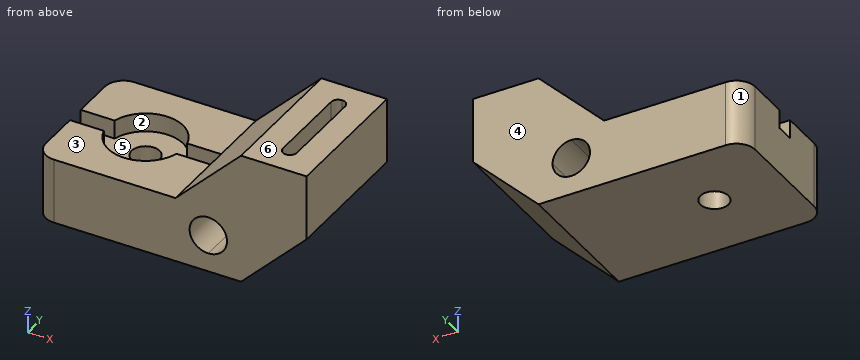
from build123d import *

# Parameters (mm, degrees)
F1_DEPTH = 76.2
F3_DEPTH = 177.8
F5_DEPTH = 27.94
F7_DEPTH = 10.16
F8_R     = 7.62
F9_DEPTH = 152.4
F10_R    = 10.16


with BuildPart() as f1:
    # F0 (on Front) → F1 (new body)
    with BuildSketch(Plane.XZ):
        Polygon((0, 35.56), (0, 0), (111.76, 0), (147.32, 35.56), (147.32, 71.12), (111.76, 71.12), (76.2, 35.56), align=None)
    extrude(amount=F1_DEPTH)

    # F2 (on face) → F3 (cut)
    with BuildSketch(Plane.XZ.offset(76.2)):
        with BuildLine():
            ThreePointArc((104.14, 20.32), (101.1642048969, 27.5042048969), (93.98, 30.48))
            Line((93.98, 30.48), (93.98, 20.32))
            Line((93.98, 20.32), (93.98, 10.16))
            ThreePointArc((93.98, 10.16), (101.1642048969, 13.1357951031), (104.14, 20.32))
        make_face()
        with BuildLine():
            Line((93.98, 20.32), (93.98, 30.48))
            ThreePointArc((93.98, 30.48), (83.82, 20.32), (93.98, 10.16))
            Line((93.98, 10.16), (93.98, 20.32))
        make_face()
    extrude(amount=-F3_DEPTH, mode=Mode.SUBTRACT)

    # F4 (on face) → F5 (cut)
    with BuildSketch(Plane.XY.offset(71.12)):
        with BuildLine():
            ThreePointArc((133.35, -15.24), (132.2340768363, -12.5459231637), (129.54, -11.43))
            Line((129.54, -11.43), (129.54, -15.24))
            Line((129.54, -15.24), (133.35, -15.24))
        make_face()
        with BuildLine():
            Line((129.54, -15.24), (129.54, -11.43))
            ThreePointArc((129.54, -11.43), (126.8459231637, -12.5459231637), (125.73, -15.24))
            Line((125.73, -15.24), (129.54, -15.24))
        make_face()
        with BuildLine():
            Line((133.35, -15.24), (129.54, -15.24))
            Line((129.54, -15.24), (129.54, -19.05))
            ThreePointArc((129.54, -19.05), (132.2340768363, -17.9340768363), (133.35, -15.24))
        make_face()
        with BuildLine():
            Line((129.54, -19.05), (129.54, -15.24))
            Line((129.54, -15.24), (125.73, -15.24))
            ThreePointArc((125.73, -15.24), (126.8459231637, -17.9340768363), (129.54, -19.05))
        make_face()
        with BuildLine():
            Line((133.35, -60.96), (133.35, -15.24))
            ThreePointArc((133.35, -15.24), (132.2340768363, -17.9340768363), (129.54, -19.05))
            Line((129.54, -19.05), (129.54, -57.15))
            ThreePointArc((129.54, -57.15), (132.2340768363, -58.2659231637), (133.35, -60.96))
        make_face()
        with BuildLine():
            ThreePointArc((129.54, -19.05), (126.8459231637, -17.9340768363), (125.73, -15.24))
            Line((125.73, -15.24), (125.73, -60.96))
            ThreePointArc((125.73, -60.96), (126.8459231637, -58.2659231637), (129.54, -57.15))
            Line((129.54, -57.15), (129.54, -19.05))
        make_face()
        with BuildLine():
            Line((129.54, -60.96), (133.35, -60.96))
            ThreePointArc((133.35, -60.96), (132.2340768363, -58.2659231637), (129.54, -57.15))
            Line((129.54, -57.15), (129.54, -60.96))
        make_face()
        with BuildLine():
            ThreePointArc((129.54, -64.77), (132.2340768363, -63.6540768363), (133.35, -60.96))
            Line((133.35, -60.96), (129.54, -60.96))
            Line((129.54, -60.96), (129.54, -64.77))
        make_face()
        with BuildLine():
            Line((129.54, -60.96), (125.73, -60.96))
            ThreePointArc((125.73, -60.96), (126.8459231637, -63.6540768363), (129.54, -64.77))
            Line((129.54, -64.77), (129.54, -60.96))
        make_face()
        with BuildLine():
            ThreePointArc((129.54, -57.15), (126.8459231637, -58.2659231637), (125.73, -60.96))
            Line((125.73, -60.96), (129.54, -60.96))
            Line((129.54, -60.96), (129.54, -57.15))
        make_face()
    extrude(amount=-F5_DEPTH, mode=Mode.SUBTRACT)

    # F6 (on face) → F7 (cut)
    with BuildSketch(Plane.XY.offset(35.56)):
        with BuildLine():
            Line((18.4252446013, -33.02), (0, -33.02))
            Line((0, -33.02), (0, -38.1))
            Line((0, -38.1), (17.78, -38.1))
            ThreePointArc((17.78, -38.1), (17.9419565719, -35.5395927768), (18.4252446013, -33.02))
        make_face()
        with BuildLine():
            Line((17.78, -38.1), (0, -38.1))
            Line((0, -38.1), (0, -43.18))
            Line((0, -43.18), (18.4252446013, -43.18))
            ThreePointArc((18.4252446013, -43.18), (17.9419565719, -40.6604072232), (17.78, -38.1))
        make_face()
        with BuildLine():
            ThreePointArc((57.7747553987, -33.02), (38.1, -17.78), (18.4252446013, -33.02))
            Line((18.4252446013, -33.02), (57.7747553987, -33.02))
        make_face()
        with BuildLine():
            Line((57.7747553987, -33.02), (18.4252446013, -33.02))
            ThreePointArc((18.4252446013, -33.02), (17.9419565719, -35.5395927768), (17.78, -38.1))
            Line((17.78, -38.1), (58.42, -38.1))
            ThreePointArc((58.42, -38.1), (58.2580434281, -35.5395927768), (57.7747553987, -33.02))
        make_face()
        with BuildLine():
            Line((58.42, -38.1), (17.78, -38.1))
            ThreePointArc((17.78, -38.1), (17.9419565719, -40.6604072232), (18.4252446013, -43.18))
            Line((18.4252446013, -43.18), (57.7747553987, -43.18))
            ThreePointArc((57.7747553987, -43.18), (58.2580434281, -40.6604072232), (58.42, -38.1))
        make_face()
        with BuildLine():
            Line((76.2, -33.02), (57.7747553987, -33.02))
            ThreePointArc((57.7747553987, -33.02), (58.2580434281, -35.5395927768), (58.42, -38.1))
            Line((58.42, -38.1), (76.2, -38.1))
            Line((76.2, -38.1), (76.2, -33.02))
        make_face()
        with BuildLine():
            Line((57.7747553987, -43.18), (18.4252446013, -43.18))
            ThreePointArc((18.4252446013, -43.18), (38.1, -58.42), (57.7747553987, -43.18))
        make_face()
        with BuildLine():
            Line((76.2, -38.1), (58.42, -38.1))
            ThreePointArc((58.42, -38.1), (58.2580434281, -40.6604072232), (57.7747553987, -43.18))
            Line((57.7747553987, -43.18), (76.2, -43.18))
            Line((76.2, -43.18), (76.2, -38.1))
        make_face()
    extrude(amount=-F7_DEPTH, mode=Mode.SUBTRACT)

    # F8 (on face) → F9 (cut)
    with BuildSketch(Plane.XY.offset(25.4)):
        with Locations((38.1, -38.1)):
            Circle(F8_R)
    extrude(amount=-F9_DEPTH, mode=Mode.SUBTRACT)

    # F10
    f10_edges = [f1.edges().sort_by_distance(p)[0] for p in [
        (0, -76.2, 17.78),
        (0, 0, 17.78),
    ]]
    fillet(f10_edges, radius=F10_R)


solid = f1.part
Input: part model. Units: mm. Frame: model coordinates. Face numbers are marked on the shaded views. A direction names the side the tool comes from. Round coordinates to 2 decimals unless told otherwise and drop trailing zeros. Loops run counter-clockwise (first coordinate to the right, second up) from the corner with the lowest first, then second, coordinate; pieces in that order, holes last. Notation, with made-up numbers: (-12, -33.75) -> (22, -33.75) arc R19 cw to (22, -11.75) -> close; hole circle Ø9 at (3.25, -9). An arc over 180 degrees is marked (long way). Answer as a JSON object with one key per item and string values. Group by question number.
1) Section query C-C on y = -20. Output: boundary loops of the cut face in (x, z), plus the area to 3 significant figures.
2) Section query D-D on z = 29. Output: boundary loops of the cut face in (x, y).
3) Draft query along Y for the marked faces 4, 5 and 6. Return one class per face: +Y half, -Y half, draft (parallel to the pull), parting line (faces both ways), or undercut.
4) Reachability of the marked faces 1, 2 and 3 from +Z, -Z, +X, -X, +Y, -Y: full face, straight path, thin tool, end or side. Return the list, or none.
5) Section query A-A on y = -38.1. Output: boundary loops of the cut face in (x, z), plus the area to 3 significant figures.
6) Pin query (flat end, axial travel): pin 1 (1 mm diameter, centred on x = 78, y = -32, fed in from -Z); pin 2 (1.5 mm diameter, centred on x = 129.5, y = -18.5, fed in from -Z); pin 3 (16.5 mm diameter, centred on x = 39.5, y = -23.5, fed in from +Z); pin 4 (2.5 mm diameter, centred on x = 128.5, y = -35, fed in from +Z). Return the tip coordinate at first contact, or that it passes through.
7) Ray query, L1, parallel to Y at x = 38, z = 5; L2, parallel to X at y = -38, z = 12; L3, parallel to Z at x = 31, y = -30. Return the intervals inside material, ascending.
8) Section query B-B on x = 38.1. Output: boundary loops of the cut face in (y, z), plus the area to 3 significant figures.
Reply:
{
 "1": {"outline": "(0, 0) -> (111.76, 0) -> (147.32, 35.56) -> (147.32, 71.12) -> (133.35, 71.12) -> (133.35, 43.18) -> (125.73, 43.18) -> (125.73, 71.12) -> (111.76, 71.12) -> (76.2, 35.56) -> (47.34, 35.56) -> (47.34, 25.4) -> (28.86, 25.4) -> (28.86, 35.56) -> (0, 35.56) -> close; hole circle Ø20.32 at (93.98, 20.32)", "area": "5,780 mm2"},
 "2": {"outline": "(0, -66.04) arc R10.16 ccw to (10.16, -76.2) -> (88.7, -76.2) -> (88.7, 0) -> (10.16, 0) arc R10.16 ccw to (0, -10.16) -> (0, -33.02) -> (18.43, -33.02) arc R20.32 cw to (57.77, -33.02) -> (76.2, -33.02) -> (76.2, -43.18) -> (57.77, -43.18) arc R20.32 cw to (18.43, -43.18) -> (0, -43.18) -> close; (99.26, -76.2) -> (140.76, -76.2) -> (140.76, 0) -> (99.26, 0) -> close"},
 "3": {"face 4": "+Y half", "face 5": "undercut", "face 6": "draft"},
 "4": {"face 1": "+Z, -Z, -X, +Y", "face 2": "+Z", "face 3": "+Z, -X, +Y, -Y"},
 "5": {"outline": "(0, 0) -> (30.48, 0) -> (30.48, 25.4) -> (0, 25.4) -> close; (45.72, 0) -> (111.76, 0) -> (147.32, 35.56) -> (147.32, 71.12) -> (133.35, 71.12) -> (133.35, 43.18) -> (125.73, 43.18) -> (125.73, 71.12) -> (111.76, 71.12) -> (76.2, 35.56) -> (76.2, 25.4) -> (45.72, 25.4) -> close; hole circle Ø20.32 at (93.98, 20.32)", "area": "4,800 mm2"},
 "6": {"pin 1": "stops at z = 0", "pin 2": "stops at z = 16.99", "pin 3": "stops at z = 35.56", "pin 4": "stops at z = 43.18"},
 "7": {"L1": "y = -76.2 to -45.72, -30.48 to 0", "L2": "x = 0 to 30.48, 45.72 to 88.15, 99.81 to 123.76", "L3": "z = 0 to 25.4"},
 "8": {"outline": "(-76.2, 0) -> (-45.72, 0) -> (-45.72, 25.4) -> (-58.42, 25.4) -> (-58.42, 35.56) -> (-76.2, 35.56) -> close; (-30.48, 0) -> (0, 0) -> (0, 35.56) -> (-17.78, 35.56) -> (-17.78, 25.4) -> (-30.48, 25.4) -> close", "area": "1,910 mm2"}
}
